Verification items for the finished model (mm, model axes). Coordinates: 2 decimals unless noted, no trailing zeros. Order: outer loops, then holes, each group sorted by start corner. A loop starts at its lowest first (then second) coordinate and runs counter-clockwise, first axis right, second up. Notation, with made-up numbers: (31, 9) -> (51, 9) arc R38 ccw to (51, 47) -> close; hole circle Ø6 at (56, 17). An arc over 180 degrees is marked (long way). Write item = value, one per line. Start each with the question number.
1. Cross-section at A-A on z = -18. Record the cut outline in (x, y), plus the area to 3 significant figures.
2. Go/stop test with flat-tipped pins: P1, Ø1.5, axis at y = 1.5, z = 19, coming from the -X side; P2, Ø0.9, axis at y = 1.5, z = 15.5, coming from the +X side. Record where each tip stops, or that it passes through.
3. Cross-section at D-D on z = -1. Record the cut outline in (x, y), plus the area to 3 significant figures.
4. Cross-section at C-C on x = 13.5. Record the cut outline in (y, z), plus the area to 3 significant figures.
5. Thickness scan on line 1 along Z through (x, y) = (0, 1.85) (3 decimals); line 2 along X through (y, z) = (1.75, 9.5); line 3 along Z through (x, y) = (-2.5, 1.25) (3 decimals). Record the ranges inside material, lowest first. Write a range as from..to.
6. Cross-section at B-B on x = 0. Record the cut outline in (y, z) (3 decimals).
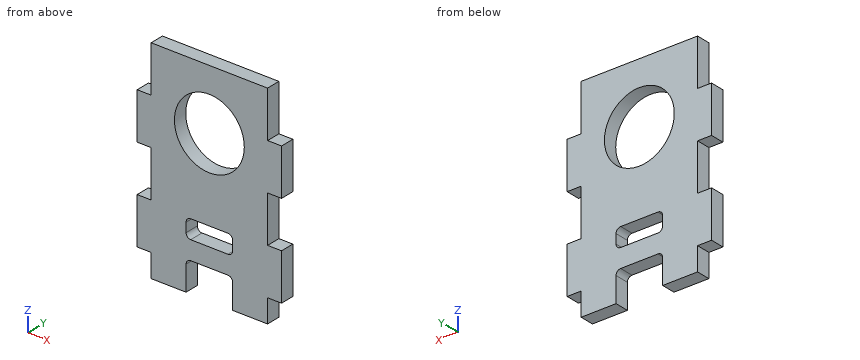
from build123d import *

# Parameters (mm, degrees)
SKETCH1_W           = 25
SKETCH1_H           = 45
BOSS_EXTRUDE1_DEPTH = 3
SKETCH2_R           = 7.5
SKETCH2_W           = 10
SKETCH2_H           = 6.365
SKETCH2_H_2         = 4
CUT_EXTRUDE1_DEPTH  = 4
FILLET1_R           = 1
SKETCH3_W           = 3
SKETCH3_H           = 10
BOSS_EXTRUDE2_DEPTH = 3


with BuildPart() as part:
    # Sketch1 → Boss-Extrude1 (new body)
    with BuildSketch(Plane(origin=(0, 0, 0), x_dir=(1, 0, 0), z_dir=(0, 1, 0))):
        Rectangle(SKETCH1_W, SKETCH1_H)
    extrude(amount=BOSS_EXTRUDE1_DEPTH)

    # Sketch2 → Cut-Extrude1 (cut, through all)
    with BuildSketch(Plane(origin=(0, 3, 0), x_dir=(1, 0, 0), z_dir=(0, 1, 0))):
        with Locations((0, -9.5)):
            Circle(SKETCH2_R)
        with Locations((0, 19.3175)):
            Rectangle(SKETCH2_W, SKETCH2_H)
        with Locations((0, 10.135)):
            Rectangle(SKETCH2_W, SKETCH2_H_2)
    extrude(amount=-CUT_EXTRUDE1_DEPTH, mode=Mode.SUBTRACT)

    # Fillet1
    fillet1_edges = [part.edges().sort_by_distance(p)[0] for p in [
        (-5, 1.5, -16.135),
        (5, 1.5, -16.135),
        (-5, 1.5, -8.135),
        (-5, 1.5, -12.135),
        (5, 1.5, -12.135),
        (5, 1.5, -8.135),
    ]]
    fillet(fillet1_edges, radius=FILLET1_R)

    # Sketch3 → Boss-Extrude2 (add)
    with BuildSketch(Plane(origin=(0, 3, 0), x_dir=(1, 0, 0), z_dir=(0, 1, 0))):
        with Locations((14, -7.5)):
            Rectangle(SKETCH3_W, SKETCH3_H)
        with Locations((14, 12.5)):
            Rectangle(SKETCH3_W, SKETCH3_H)
        with Locations((-14, -7.5)):
            Rectangle(SKETCH3_W, SKETCH3_H)
        with Locations((-14, 12.5)):
            Rectangle(SKETCH3_W, SKETCH3_H)
    extrude(amount=-BOSS_EXTRUDE2_DEPTH)


solid = part.part
Worked out:
q1.outline = (-12.5, 0) -> (-5, 0) -> (-5, 3) -> (-12.5, 3) -> close; (5, 0) -> (12.5, 0) -> (12.5, 3) -> (5, 3) -> close
q1.area = 45.0 mm²
q2.P1 = -12.5
q2.P2 = 12.5
q3.outline = (-12.5, 0) -> (12.5, 0) -> (12.5, 3) -> (-12.5, 3) -> close
q3.area = 75.0 mm²
q4.outline = (0, -17.5) -> (3, -17.5) -> (3, -7.5) -> (0, -7.5) -> close; (0, 2.5) -> (3, 2.5) -> (3, 12.5) -> (0, 12.5) -> close
q4.area = 60.0 mm²
q5.line_1 = -16.135..-12.135, -8.135..2, 17..22.5
q5.line_2 = -15.5..-7.5, 7.5..15.5
q5.line_3 = -16.135..-12.135, -8.135..2.429, 16.571..22.5
q6.outline = (0, -16.135) -> (3, -16.135) -> (3, -12.135) -> (0, -12.135) -> close; (0, -8.135) -> (3, -8.135) -> (3, 2) -> (0, 2) -> close; (0, 17) -> (3, 17) -> (3, 22.5) -> (0, 22.5) -> close
